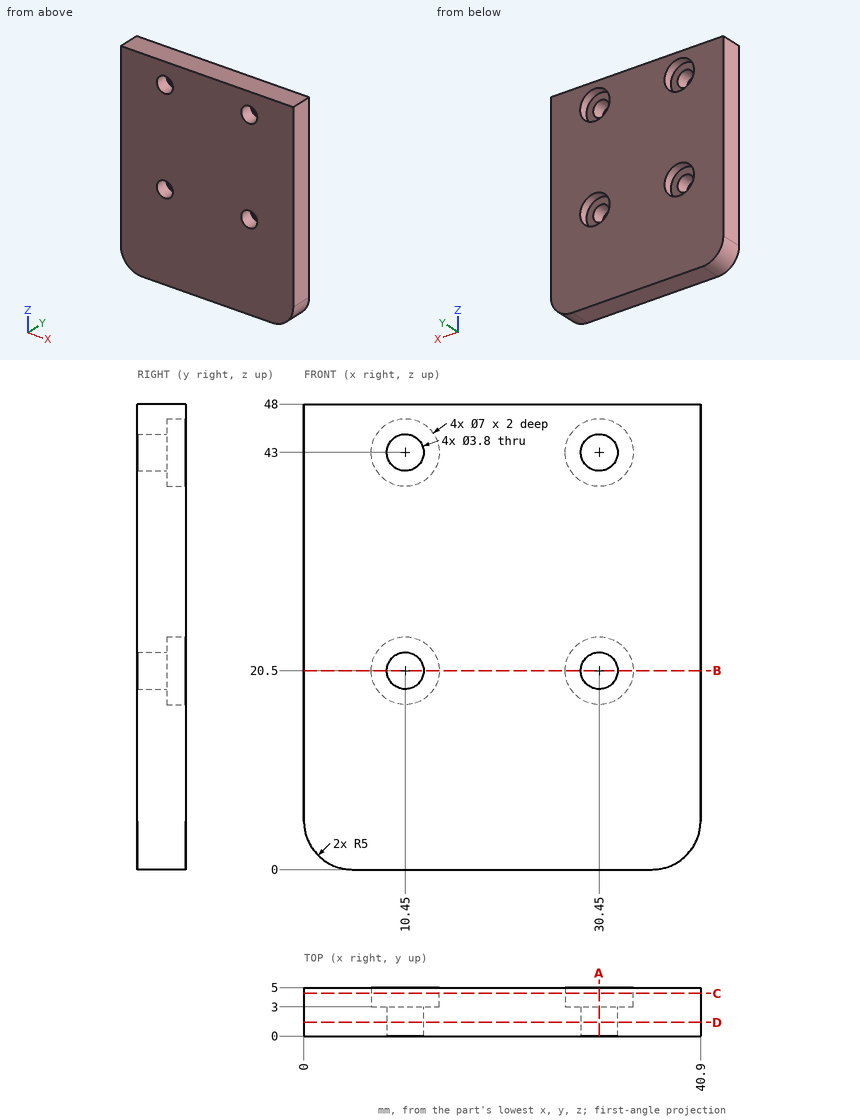
Could you check a few things on this drawing? It's one solid part, dimensions in mm from its lowest x, y, z. Round coordinates to 2 decimals unless told otherwise and drop trailing zeros. Order: outer loops, then holes, each group sorted by start corner. A loop starts at its lowest first (then second) coordinate and runs counter-clockwise, first axis right, second up. Notation, with made-up numbers: M 14,-23.75 L 43,-23.75 A31 cw 43,0.25 Z; hole C -6,41.25 d1. An arc over 180 degrees is marked long. One line per question, with ' | ' between items. Start each with the question number.
(1) Please list where these lines run through material, in increasing order: line 1 along Z through (x, y) = (10.45, 3.7); line 2 along Z through (x, y) = (10.45, 0.85); line 3 along X through (y, z) = (1.45, 41.5).
(2) Suppose I cut it at D-D on y = 1.4. List the corners of the cut face in (x, z) for me, then the cut area to 3 significant figures.
(3) Suppose I cut it at C-C on y = 4.4. List the corners of the cut face in (x, z) for me.
(4) Suppose I cut it at B-B on z = 20.5. List the corners of the cut face in (x, y) for me.
(5) For P1, Ø5.5, axis at x = 10, z = 42.5, coming from the +Y side, with a flat end and sliding along its axis, tell me the tip position at first contact or that it passes through.
(6) Suppose I cut it at A-A on x = 30.45. List the corners of the cut face in (y, z) for me, then the cut area to 3 significant figures.
Geometry results:
1) line 1: 0 to 17, 24 to 39.5, 46.5 to 48 | line 2: 0 to 18.6, 22.4 to 41.1, 44.9 to 48 | line 3: 0 to 9.28, 11.62 to 29.28, 31.62 to 40.9
2) outline: M 0,5 A5 ccw 5,0 L 35.9,0 A5 ccw 40.9,5 L 40.9,48 L 0,48 Z; hole C 10.45,20.5 d3.8; hole C 10.45,43 d3.8; hole C 30.45,20.5 d3.8; hole C 30.45,43 d3.8 | area: 1,910 mm²
3) outline: M 0,5 A5 ccw 5,0 L 35.9,0 A5 ccw 40.9,5 L 40.9,48 L 0,48 Z; hole C 10.45,20.5 d7; hole C 10.45,43 d7; hole C 30.45,20.5 d7; hole C 30.45,43 d7
4) outline: M 0,0 L 8.55,0 L 8.55,3 L 6.95,3 L 6.95,5 L 0,5 Z; M 12.35,0 L 28.55,0 L 28.55,3 L 26.95,3 L 26.95,5 L 13.95,5 L 13.95,3 L 12.35,3 Z; M 32.35,0 L 40.9,0 L 40.9,5 L 33.95,5 L 33.95,3 L 32.35,3 Z
5) P1: y = 3
6) outline: M 0,0 L 5,0 L 5,17 L 3,17 L 3,18.6 L 0,18.6 Z; M 0,22.4 L 3,22.4 L 3,24 L 5,24 L 5,39.5 L 3,39.5 L 3,41.1 L 0,41.1 Z; M 0,44.9 L 3,44.9 L 3,46.5 L 5,46.5 L 5,48 L 0,48 Z | area: 189 mm²
